The drawing under review shows one solid part. Ordinate dimensions are in mm from its lowest x, y, z. A direction names the side the tool comes from. Coordinates: 2 decimals unless noted, no trailing zeros. Order: outer loops, then holes, each group sorted by start corner. A loop starts at its lowest first (then second) coordinate and runs counter-clockwise, first axis right, second up.
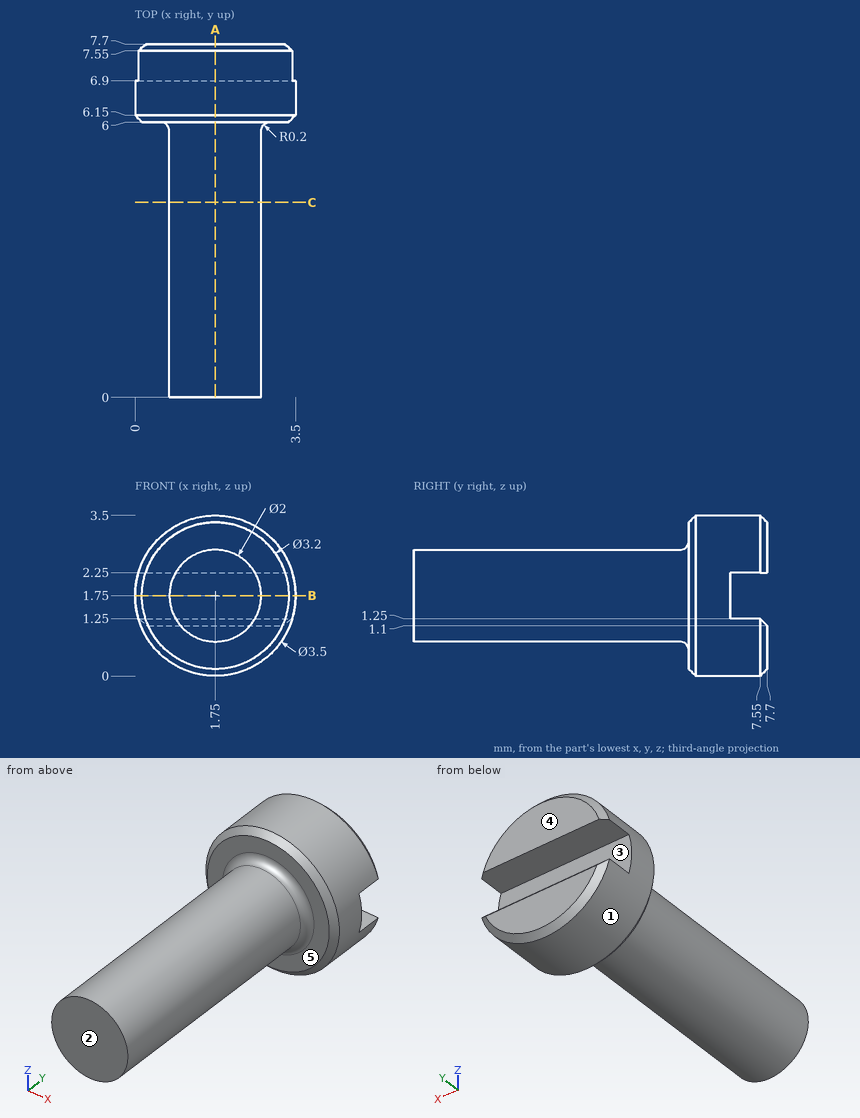
1. Take a section at A-A, the plane x = 1.75. Give the boundary of the cut face in (y, z), plus the area to 3 significant figures.
Answer below:
outline: (0, 0.75) - (5.8, 0.75) arc R0.2 cw to (6, 0.55) - (6, 0.15) - (6.15, 0) - (7.55, 0) - (7.7, 0.15) - (7.7, 1.1) - (7.55, 1.25) - (6.9, 1.25) - (6.9, 2.25) - (7.7, 2.25) - (7.7, 3.35) - (7.55, 3.5) - (6.15, 3.5) - (6, 3.35) - (6, 2.95) arc R0.2 cw to (5.8, 2.75) - (0, 2.75) - close
area: 17.1 mm2
2. To check wall thickness, follow L1, parallel to X at y = 5.25, z = 1.7; L2, parallel to Y at x = 0.5, z = 1.45; L3, parallel to Y at x = 2.6, z = 1.3. State the ranges of each line that lie inside material, in increasing order.
Answer below:
L1: x = 0.75 to 2.75
L2: y = 6 to 6.9
L3: y = 0 to 6.9
3. Take a section at C-C, the plane y = 4.25. Give the boundary of the cut face in (x, z), plus the area to 3 significant figures.
Answer below:
outline: circle Ø2 at (1.75, 1.75)
area: 3.14 mm2
4. Machinability: for the marked faces 4 and 5, which of the approach directions +Z, -Z, +X, -X, +Y, -Y give a long, thin tool a straight path to every point of the face, cutting with its end or side? Answer none if there is none.
Answer below:
face 4: +Z, -Z, +X, -X, +Y
face 5: -Y
5. Clearance check with flat-ended pins moving along their axes: pin 1 Ø1 at (x, y) = (1.5, 4) entering from -Z; pin 2 Ø1.5 at (x, y) = (0.5, 2) entering from -Z. State where each tip first meets the part, or that it passes through.
Answer below:
pin 1: stops at z = 0.75
pin 2: stops at z = 0.88
6. Take a section at B-B, the plane z = 1.75. Give the boundary of the cut face in (x, y).
Answer below:
outline: (0, 6.15) - (0.15, 6) - (0.55, 6) arc R0.2 cw to (0.75, 5.8) - (0.75, 0) - (2.75, 0) - (2.75, 5.8) arc R0.2 cw to (2.95, 6) - (3.35, 6) - (3.5, 6.15) - (3.5, 6.9) - (0, 6.9) - close
7. The part is to be moulded in two halves that separate along Z. For the marked faces 1, 2 and 3, say which applies: +Z half, -Z half, draft (parallel to the pull), parting line (faces both ways), or undercut.
Answer below:
face 1: parting line
face 2: draft
face 3: undercut
